The listing builds one solid part. Answer for the finished solid, in the listing's coordinates (mm). A direction names the side the tool comes from. Coordinates: 2 decimals unless noted, no trailing zeros. Loops run counter-clockwise (first coordinate to the right, second up) from the corner with the lowest first, then second, coordinate; pieces in that order, holes last. Notation, with made-up numbers: (68.25, 52) - (113.25, 52) arc R9 cw to (113.25, 65) - close; hole circle Ø2 at (45.5, 46.25). An arc over 180 degrees is marked (long way). Return JSON: item names as keys, results as strings. Group by question number.
1. Each of these flat-tipped pins is pushed along its axis until it touches: P1, Ø3, axis at x = 9, z = -11.5, coming from the +Y side; P2, Ø1.8, axis at x = -10.5, z = -11, coming from the -Y side; P3, Ø3, axis at y = 10, z = -11.5, coming from the -X side. Where does it stop, or does it pass through?
2. Section D-D (z = 8.25) is taken. Write down the section's boundary in (x, y).
3. Section A-A (z = -7.75) is taken. Write down the section's boundary in (x, y) (3 decimals), and give its area (3 significant figures).
4. Which of the six approach directions +Z, -Z, +X, -X, +Y, -Y give full straight-line access (tool end or side, diameter ignored) to faces 1 (the face through (8, -23, -7)), 2 (the face through (17.85, -4.69, -11.18)), 3 (the face through (-2.831, 21.565, -0.022)), 4 (the face through (-22, -14, 13))?
5. Find the intervals of material crossed by line 1 along Y through (x, z) = (0, -11.95); line 2 along Y through (x, z) = (0, -2.75) (3 decimals); line 3 along Z through (x, y) = (-22.5, 11), in increasing order.
6. Section B-B (y = 0) is taken. State how many separate pieces and enclosed holes the cut face has, and give its area (3 significant figures).
7. The mould has two halves that part along Z. Classify faces 5 (the face through (0, 0, -13)), 6 (the face through (-4, 11, -11)), 7 (the face through (-8, -23, 7)): pulls with the +Z half, pulls with the -Z half, needs draft (parallel to the pull), parting line crosses it, or undercut.
```python
from build123d import *

# Parameters (mm, degrees)
SKETCH_3_R          = 21.75
CUT_EXTRUDE_1_DEPTH = 22.3
FILLET_1_R          = 4
CUT_EXTRUDE_3_REACH = 45.61
SKETCH_4_R          = 1.35
SKETCH_6_R          = 2.975
EXTRUDE_2_DEPTH     = 15.5
FILLET_2_R          = 2


with BuildPart() as part:
    # Sketch 1 → Revolve 1 (revolve)
    with BuildSketch(Plane(origin=(0, 0, 0), x_dir=(0, 0, -1), z_dir=(1, 0, 0)), mode=Mode.PRIVATE) as revolve_1_sk:
        Polygon((-5, 24), (5, 24), (7, 25.6), (7, 24), (10.5, 24), (10.5, 26.5), (13, 26.5), (13, 0), (-13, 0), (-13, 26.5), (-10.5, 26.5), (-10.5, 24), (-7, 24), (-7, 25.6), align=None)
    revolve(revolve_1_sk.sketch.rotate(Axis((0, 0, -13), (0, 0, 1)), 90), axis=Axis((0, 0, -13), (0, 0, 1)))

    # Sketch 3 → Cut-Extrude 1 (cut)
    with BuildSketch(Plane.XY.offset(13)):
        Circle(SKETCH_3_R)
    extrude(amount=-CUT_EXTRUDE_1_DEPTH, mode=Mode.SUBTRACT)

    # Fillet 1
    fillet_1_edges = [part.edges().sort_by_distance(p)[0] for p in [
        (-21.75, 0, 13),
    ]]
    fillet(fillet_1_edges, radius=FILLET_1_R)

    # Sketch 4 → Cut-Extrude 3 (cut, up to next)
    with BuildSketch(Plane.XY.offset(-9.3), mode=Mode.PRIVATE) as cut_extrude_3_sk1:
        with Locations((8, 0)):
            Circle(SKETCH_4_R)
    cut_extrude_3_tool1 = extrude(cut_extrude_3_sk1.sketch, amount=-CUT_EXTRUDE_3_REACH, mode=Mode.PRIVATE) & part.part
    # Sketch 4 → Cut-Extrude 3 (cut, up to next)
    with BuildSketch(Plane.XY.offset(-9.3), mode=Mode.PRIVATE) as cut_extrude_3_sk2:
        with BuildLine():
            Line((-18.5, 4), (-4, 4))
            Line((-4, 4), (-4, 18.5))
            ThreePointArc((-4, 18.5), (-14.253048327, 14.253048327), (-18.5, 4))
        make_face()
    cut_extrude_3_tool2 = extrude(cut_extrude_3_sk2.sketch, amount=-CUT_EXTRUDE_3_REACH, mode=Mode.PRIVATE) & part.part
    # Sketch 4 → Cut-Extrude 3 (cut, up to next)
    with BuildSketch(Plane.XY.offset(-9.3), mode=Mode.PRIVATE) as cut_extrude_3_sk3:
        with BuildLine():
            Line((4, 18.5), (4, 4))
            Line((4, 4), (18.5, 4))
            ThreePointArc((18.5, 4), (14.253048327, 14.253048327), (4, 18.5))
        make_face()
    cut_extrude_3_tool3 = extrude(cut_extrude_3_sk3.sketch, amount=-CUT_EXTRUDE_3_REACH, mode=Mode.PRIVATE) & part.part
    # Sketch 4 → Cut-Extrude 3 (cut, up to next)
    with BuildSketch(Plane.XY.offset(-9.3), mode=Mode.PRIVATE) as cut_extrude_3_sk4:
        with BuildLine():
            Line((18.5, -4), (4, -4))
            Line((4, -4), (4, -18.5))
            ThreePointArc((4, -18.5), (14.253048327, -14.253048327), (18.5, -4))
        make_face()
    cut_extrude_3_tool4 = extrude(cut_extrude_3_sk4.sketch, amount=-CUT_EXTRUDE_3_REACH, mode=Mode.PRIVATE) & part.part
    # Sketch 4 → Cut-Extrude 3 (cut, up to next)
    with BuildSketch(Plane.XY.offset(-9.3), mode=Mode.PRIVATE) as cut_extrude_3_sk5:
        with BuildLine():
            Line((-4, -18.5), (-4, -4))
            Line((-4, -4), (-18.5, -4))
            ThreePointArc((-18.5, -4), (-14.253048327, -14.253048327), (-4, -18.5))
        make_face()
    cut_extrude_3_tool5 = extrude(cut_extrude_3_sk5.sketch, amount=-CUT_EXTRUDE_3_REACH, mode=Mode.PRIVATE) & part.part
    # Sketch 4 → Cut-Extrude 3 (cut, up to next)
    with BuildSketch(Plane.XY.offset(-9.3), mode=Mode.PRIVATE) as cut_extrude_3_sk6:
        with Locations((0, -8)):
            Circle(SKETCH_4_R)
    cut_extrude_3_tool6 = extrude(cut_extrude_3_sk6.sketch, amount=-CUT_EXTRUDE_3_REACH, mode=Mode.PRIVATE) & part.part
    # Sketch 4 → Cut-Extrude 3 (cut, up to next)
    with BuildSketch(Plane.XY.offset(-9.3), mode=Mode.PRIVATE) as cut_extrude_3_sk7:
        with Locations((-8, 0)):
            Circle(SKETCH_4_R)
    cut_extrude_3_tool7 = extrude(cut_extrude_3_sk7.sketch, amount=-CUT_EXTRUDE_3_REACH, mode=Mode.PRIVATE) & part.part
    # Sketch 4 → Cut-Extrude 3 (cut, up to next)
    with BuildSketch(Plane.XY.offset(-9.3), mode=Mode.PRIVATE) as cut_extrude_3_sk8:
        with Locations((0, 8)):
            Circle(SKETCH_4_R)
    cut_extrude_3_tool8 = extrude(cut_extrude_3_sk8.sketch, amount=-CUT_EXTRUDE_3_REACH, mode=Mode.PRIVATE) & part.part
    add(cut_extrude_3_tool1.solids().sort_by_distance((8, 0, -9.3))[0], mode=Mode.SUBTRACT)
    add(cut_extrude_3_tool2.solids().sort_by_distance((-10.153991, 10.153991, -9.3))[0], mode=Mode.SUBTRACT)
    add(cut_extrude_3_tool3.solids().sort_by_distance((10.153991, 10.153991, -9.3))[0], mode=Mode.SUBTRACT)
    add(cut_extrude_3_tool4.solids().sort_by_distance((10.153991, -10.153991, -9.3))[0], mode=Mode.SUBTRACT)
    add(cut_extrude_3_tool5.solids().sort_by_distance((-10.153991, -10.153991, -9.3))[0], mode=Mode.SUBTRACT)
    add(cut_extrude_3_tool6.solids().sort_by_distance((0, -8, -9.3))[0], mode=Mode.SUBTRACT)
    add(cut_extrude_3_tool7.solids().sort_by_distance((-8, 0, -9.3))[0], mode=Mode.SUBTRACT)
    add(cut_extrude_3_tool8.solids().sort_by_distance((0, 8, -9.3))[0], mode=Mode.SUBTRACT)

    # Sketch 6 → Extrude 2 (add)
    with BuildSketch(Plane.XY.offset(-9.3)):
        Circle(SKETCH_6_R)
    extrude(amount=EXTRUDE_2_DEPTH)

    # Fillet 2
    fillet_2_edges = [part.edges().sort_by_distance(p)[0] for p in [
        (18.5, 4, -11.15),
        (4, 4, -11.15),
        (4, 18.5, -11.15),
        (18.5, -4, -11.15),
        (4, -18.5, -11.15),
        (4, -4, -11.15),
        (-18.5, -4, -11.15),
        (-4, -4, -11.15),
        (-4, -18.5, -11.15),
        (-18.5, 4, -11.15),
        (-4, 18.5, -11.15),
        (-4, 4, -11.15),
    ]]
    fillet(fillet_2_edges, radius=FILLET_2_R)


solid = part.part
```
The answers:
{
 "1": {"P1": "stops at y = 25.42", "P2": "stops at y = -24.7", "P3": "stops at x = -25.1"},
 "2": {"outline": "circle Ø48 at (0, 0); hole circle Ø43.5 at (0, 0)"},
 "3": {"outline": "circle Ø48 at (0, 0); circle Ø5.95 at (0, 0); hole circle Ø43.5 at (0, 0)", "area": "351 mm2"},
 "4": {"face 1": "none", "face 2": "+Z, -Z", "face 3": "+Z", "face 4": "+Z, +X, -X, +Y, -Y"},
 "5": {"line 1": "y = -26.5 to -9.35, -6.65 to 6.65, 9.35 to 26.5", "line 2": "y = -24 to -21.75, -2.975 to 2.975, 21.75 to 24", "line 3": "z = -13 to -10.5, -7 to -6.31, 6.31 to 7, 10.5 to 12.94"},
 "6": {"separate pieces": "3", "enclosed holes": "0", "area": "375 mm2"},
 "7": {"face 5": "pulls with the -Z half", "face 6": "needs draft", "face 7": "undercut"}
}
